from build123d import *

# Parameters (mm, degrees)
SKETCH1_W           = 25.4
SKETCH1_H           = 39.37
SKETCH1_R           = 1.524
BOSS_EXTRUDE1_DEPTH = 2.54
FILLET1_R           = 2.54


with BuildPart() as part:
    # Sketch1 → Boss-Extrude1 (new body)
    with BuildSketch(Plane.XY):
        with Locations((12.7, -19.685)):
            Rectangle(SKETCH1_W, SKETCH1_H)
        with Locations((4.7625, -19.685)):
            Circle(SKETCH1_R, mode=Mode.SUBTRACT)
        with Locations((20.6375, -19.685)):
            Circle(SKETCH1_R, mode=Mode.SUBTRACT)
        with Locations((4.7625, -10.795)):
            Circle(SKETCH1_R, mode=Mode.SUBTRACT)
        with Locations((20.6375, -10.795)):
            Circle(SKETCH1_R, mode=Mode.SUBTRACT)
        with Locations((4.7625, -28.575)):
            Circle(SKETCH1_R, mode=Mode.SUBTRACT)
        with Locations((20.6375, -28.575)):
            Circle(SKETCH1_R, mode=Mode.SUBTRACT)
        with Locations((12.7, -3.175)):
            Circle(SKETCH1_R, mode=Mode.SUBTRACT)
        with Locations((12.7, -36.195)):
            Circle(SKETCH1_R, mode=Mode.SUBTRACT)
    extrude(amount=BOSS_EXTRUDE1_DEPTH)

    # Fillet1
    fillet1_edges = [part.edges().sort_by_distance(p)[0] for p in [
        (0, 0, 1.27),
        (25.4, 0, 1.27),
        (25.4, -39.37, 1.27),
        (0, -39.37, 1.27),
    ]]
    fillet(fillet1_edges, radius=FILLET1_R)


solid = part.part
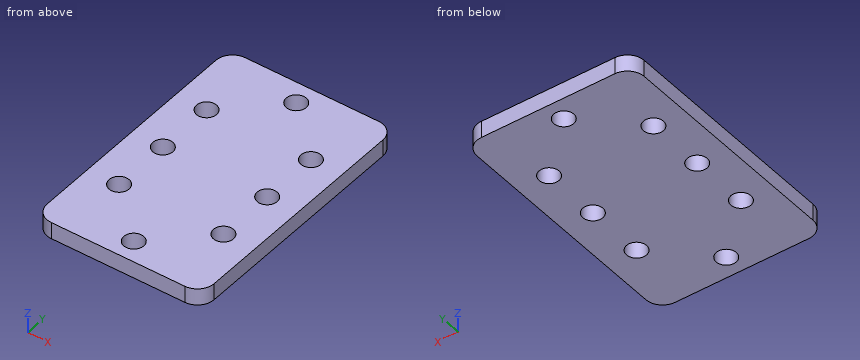
The listing builds one solid part. Answer for the finished solid, in the listing's coordinates (mm). Round coordinates to 2 decimals unless told otherwise and drop trailing zeros. Order: outer loops, then holes, each group sorted by start corner. A loop starts at its lowest first (then second) coordinate and runs counter-clockwise, first axis right, second up. Notation, with made-up numbers: (5.25, 32.5) -> (18.25, 32.5) arc R36 ccw to (18.25, 69.5) -> close; hole circle Ø1 at (30, -32.75). An arc over 180 degrees is marked (long way). Write each question's results on one line, items separated by ' | '. Start each with the question number.
Q1. Straight lines are drawn through the part: probe 1 along Y at (x, z) = (12.7, 0.65); probe 2 along Y at (x, z) = (4.75, 0.65); probe 3 along Y at (x, z) = (21.5, 2). For each, find the intervals that lie inside material, in ascending order. Write a range as from..to.
Q2. Find section A-A (x = 12.7). Determine the outline of the cut face in (y, z).
Q3. Find section C-C (x = 20). Determine the outline of the cut face in (y, z).
Q4. Find section D-D (y = -4). Determine the outline of the cut face in (x, z).
Q5. Find section B-B (z = 1.4). Give the number of separate pieces and of enclosed holes in the cut face, then the cut area to 3 significant figures.
Worked answers:
1) probe 1: y = -39.37..-37.72, -34.67..-4.7, -1.65..0 | probe 2: y = -39.37..-30.1, -27.05..-21.21, -18.16..-12.32, -9.27..0 | probe 3: y = -39.37..-29.83, -27.32..-20.94, -18.43..-12.05, -9.54..0
2) outline: (-39.37, 0) -> (-37.72, 0) -> (-37.72, 2.54) -> (-39.37, 2.54) -> close; (-34.67, 0) -> (-4.7, 0) -> (-4.7, 2.54) -> (-34.67, 2.54) -> close; (-1.65, 0) -> (0, 0) -> (0, 2.54) -> (-1.65, 2.54) -> close
3) outline: (-39.37, 0) -> (-29.96, 0) -> (-29.96, 2.54) -> (-39.37, 2.54) -> close; (-27.19, 0) -> (-21.07, 0) -> (-21.07, 2.54) -> (-27.19, 2.54) -> close; (-18.3, 0) -> (-12.18, 0) -> (-12.18, 2.54) -> (-18.3, 2.54) -> close; (-9.41, 0) -> (0, 0) -> (0, 2.54) -> (-9.41, 2.54) -> close
4) outline: (0, 0) -> (11.42, 0) -> (11.42, 2.54) -> (0, 2.54) -> close; (13.98, 0) -> (25.4, 0) -> (25.4, 2.54) -> (13.98, 2.54) -> close
5) separate pieces: 1 | enclosed holes: 8 | area: 936 mm2
